Design review of the part built by this model. Coordinates are the model's own, in mm. Face numbers are marked on the shaded views. A direction names the side the tool comes from. Round coordinates to 2 decimals unless told otherwise and drop trailing zeros. Loops run counter-clockwise (first coordinate to the right, second up) from the corner with the lowest first, then second, coordinate; pieces in that order, holes last. Notation, with made-up numbers: (8, 32.25) - (49, 32.25) arc R19 cw to (49, 54.25) - close; hole circle Ø7 at (13, -23). An arc over 180 degrees is marked (long way). Return JSON: item names as keys, results as strings. Group by question number.
from build123d import *

# Parameters (mm, degrees)
SK_CABEZA_AVELLANADA_R  = 3.75
CABEZA_AVELLANADA_DEPTH = 2.5
SK_CUERPO_R             = 2
CUERPO_DEPTH            = 16
HEXAGONO_INTERIOR_DEPTH = 1.5


with BuildPart() as part:
    # Sk_Cabeza_avellanada → Cabeza_avellanada (new body)
    with BuildSketch(Plane.XY):
        Circle(SK_CABEZA_AVELLANADA_R)
    extrude(amount=CABEZA_AVELLANADA_DEPTH)

    # Sk_Cuerpo → Cuerpo (add)
    with BuildSketch(Plane.XY):
        Circle(SK_CUERPO_R)
    extrude(amount=CUERPO_DEPTH)

    # Sk_Hexagono_interior → Hexagono_interior (cut)
    with BuildSketch(Plane.XY):
        Polygon((0, -1.443375673), (1.25, -0.721687836), (1.25, 0.721687836), (0, 1.443375673), (-1.25, 0.721687836), (-1.25, -0.721687836), align=None)
    extrude(amount=HEXAGONO_INTERIOR_DEPTH, mode=Mode.SUBTRACT)


solid = part.part
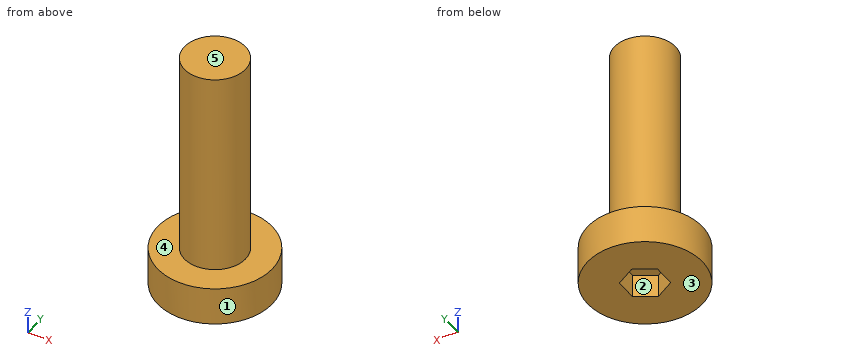
Q1. Add section A-A, the plane y = 0. State the section outline as (x, z) points, plus the area to 3 significant figures.
Q2. Add section B-B, the plane x = -1.75. State the section outline as (y, z) points, plus the area to 3 significant figures.
Q3. For line 1 (Z direction, x = -1, y = 3); line 2 (Z direction, x = -0.25, y = -1); line 3 (Y direction, x = 0, z = 9.75), list the stretches that pass through material, from the lowest coordinate up.
Q4. Add section D-D, the plane y = -3. State the section outline as (x, z) points.
Q5. Tool access review of the marked faces 4 and 5: name each direction out of +Z, -Z, +X, -X, +Y, -Y from which nothing blocks a thin tool from reaching the whole face with its end or side.
Q6. Insertion check: pin 1 Ø2 at (x, z) = (3, 3) entering from -Y; pin 2 Ø1 at (y, z) = (2, 6) entering from -X; pin 3 Ø1.5 at (x, z) = (-1.5, 1.5) entering from +Y. Each pin has a flat end and moves straight along its axis. Give the tip position at first contact, or say it passes through.
Q7. Draft analysis for pull direction X (two halves, no side actions). For the marked faces 1, 2 and 3, state which applies: pulls with the +X half, pulls with the -X half, needs draft (parallel to the pull), parting line crosses it, or undercut.
Q8. Add section C-C, the plane z = 10. State the section outline as (x, y) points, plus the area to 3 significant figures.
Evaluation:
{
 "1": {"outline": "(-3.75, 0) - (-1.25, 0) - (-1.25, 1.5) - (1.25, 1.5) - (1.25, 0) - (3.75, 0) - (3.75, 2.5) - (2, 2.5) - (2, 16) - (-2, 16) - (-2, 2.5) - (-3.75, 2.5) - close", "area": "69.0 mm²"},
 "2": {"outline": "(-3.32, 0) - (3.32, 0) - (3.32, 2.5) - (0.97, 2.5) - (0.97, 16) - (-0.97, 16) - (-0.97, 2.5) - (-3.32, 2.5) - close", "area": "42.7 mm²"},
 "3": {"line 1": "0 to 2.5", "line 2": "1.5 to 16", "line 3": "-2 to 2"},
 "4": {"outline": "(-2.25, 0) - (2.25, 0) - (2.25, 2.5) - (-2.25, 2.5) - close"},
 "5": {"face 4": "+Z", "face 5": "+Z, +X, -X, +Y, -Y"},
 "6": {"pin 1": "y = -3.08", "pin 2": "x = -1.32", "pin 3": "y = 3.67"},
 "7": {"face 1": "parting line crosses it", "face 2": "undercut", "face 3": "needs draft"},
 "8": {"outline": "circle Ø4 at (0, 0)", "area": "12.6 mm²"}
}
